Work out the finished part from the listing and answer in its coordinate system (mm). Face numbers are marked on the shaded views. A direction names the side the tool comes from. Round coordinates to 2 decimals unless told otherwise and drop trailing zeros. Write each loop counter-clockwise with the first axis right and the second up, starting at its lowest first coordinate (ties: lowest second). Pieces come first, ordered by that corner, then holes. Notation, with made-up numbers: M -26.75,73 L -7.75,73 A19 cw -7.75,93 Z; hole C 44.25,25.5 d6. An arc over 180 degrees is marked long. One line per item, written item: value. Start each with the question number.
Q1. Find section C-C (y = -2.5). Write down the section's boundary in (x, z), and give its area (3 significant figures).
Q2. Consider probe 1 along X at (y, z) = (-4.3, 0); probe 2 along Z at (x, y) = (0, -0.75). Determine where each line is inside the solid, lowest interval first.
Q3. Find section A-A (z = 0). Write down the section's boundary in (x, y), and give its area (3 significant figures).
Q4. The mould has two halves that part along X. Classify the marked faces 1 and 2: released by +X, released by -X, zero draft, split by the parting line, or undercut.
Q5. Given pin 1 Ø1.5 at (y, z) = (3.5, -9) entering from +X; pin 2 Ø3 at (x, y) = (-24, -1.5) entering from +Z; pin 3 Ø20.5 at (x, z) = (-7.5, -14.5) entering from -Y; pin 4 Ø5 at (x, y) = (16.5, 0.5) entering from -Z, each flat-ended and moving along its own axis, determine where each tip first touches the part or whether it passes through.
Q6. A tool of negligible diameter and unlimited length cuts with its end or side. For the marked faces 3 and 4, from which of +Z, -Z, +X, -X, +Y, -Y can it reach the whole face along a straight path? Write none if from no direction.
Q7. Find section B-B (x = 0). Write down the section's boundary in (y, z), and give its area (3 significant figures).
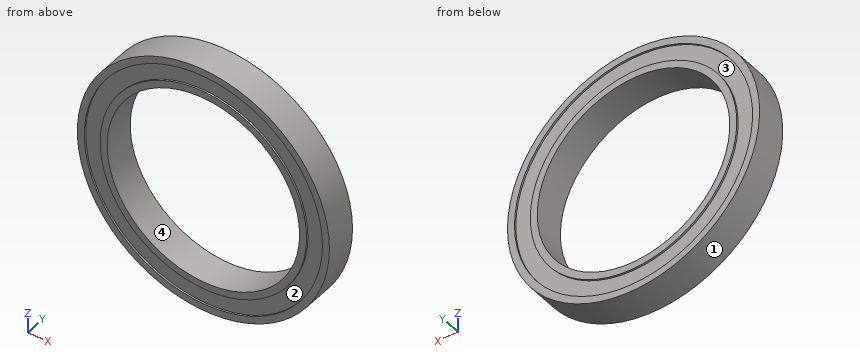
from build123d import *

# Parameters (mm, degrees)
SKETCH_1_R          = 36
SKETCH_1_R_2        = 27.5
EXTRUDE_1_DEPTH     = 4.5
SKETCH_3_R          = 34
SKETCH_3_R_2        = 29.5
CUT_EXTRUDE_1_DEPTH = 0.5


with BuildPart() as part:
    # 草图1 → 凸台-拉伸1 (new body, symmetric)
    with BuildSketch(Plane(origin=(0, 0, 0), x_dir=(1, 0, 0), z_dir=(0, 1, 0))):
        Circle(SKETCH_1_R)
        Circle(SKETCH_1_R_2, mode=Mode.SUBTRACT)
    extrude(amount=EXTRUDE_1_DEPTH, both=True)

    # 草图3 → 切除-拉伸1 (cut)
    with BuildSketch(Plane(origin=(0, 4.5, 0), x_dir=(1, 0, 0), z_dir=(0, 1, 0))):
        Circle(SKETCH_3_R)
        Circle(SKETCH_3_R_2, mode=Mode.SUBTRACT)
    cut_extrude_1 = extrude(amount=-CUT_EXTRUDE_1_DEPTH, mode=Mode.SUBTRACT)

    # 镜向1: 切除-拉伸1 across plane
    add(cut_extrude_1.mirror(Plane.ZX), mode=Mode.SUBTRACT)


solid = part.part
The answers:
1. outline: C 0,0 d72; hole C 0,0 d55
1. area: 1,700 mm2
2. probe 1: -36 to -34, -29.5 to -27.5, 27.5 to 29.5, 34 to 36
2. probe 2: -36 to -27.5, 27.5 to 36
3. outline: M -36,-4.5 L -34,-4.5 L -34,-4 L -29.5,-4 L -29.5,-4.5 L -27.5,-4.5 L -27.5,4.5 L -29.5,4.5 L -29.5,4 L -34,4 L -34,4.5 L -36,4.5 Z; M 27.5,-4.5 L 29.5,-4.5 L 29.5,-4 L 34,-4 L 34,-4.5 L 36,-4.5 L 36,4.5 L 34,4.5 L 34,4 L 29.5,4 L 29.5,4.5 L 27.5,4.5 Z
3. area: 144 mm2
4. face 1: split by the parting line
4. face 2: undercut
5. pin 1: x = 35.04
5. pin 2: z = 28.1
5. pin 3: through
5. pin 4: z = -33.17
6. face 3: +Y
6. face 4: +Y, -Y
7. outline: M -4.5,-36 L 4.5,-36 L 4.5,-34 L 4,-34 L 4,-29.5 L 4.5,-29.5 L 4.5,-27.5 L -4.5,-27.5 L -4.5,-29.5 L -4,-29.5 L -4,-34 L -4.5,-34 Z; M -4.5,27.5 L 4.5,27.5 L 4.5,29.5 L 4,29.5 L 4,34 L 4.5,34 L 4.5,36 L -4.5,36 L -4.5,34 L -4,34 L -4,29.5 L -4.5,29.5 Z
7. area: 144 mm2
